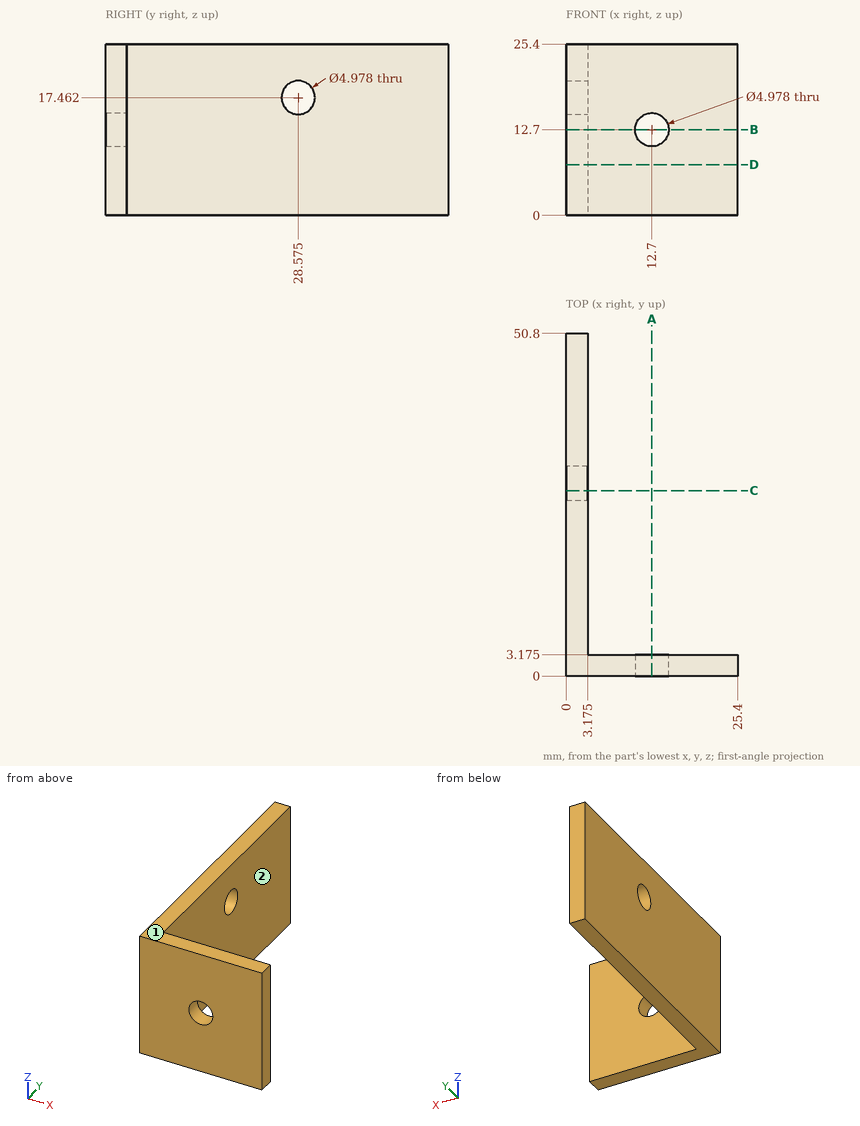
Design review of the part shown in the three views and the two pictorial views. Dimensions are in mm from the part's minimum x, y and z. A direction names the side the tool comes from. Coordinates: 2 decimals unless noted, no trailing zeros. Order: outer loops, then holes, each group sorted by start corner. A loop starts at its lowest first (then second) coordinate and runs counter-clockwise, first axis right, second up.
1) Clearance check with flat-ended pins moving along their axes: pin 1 (8 mm diameter, centred on x = 4, z = 15, fed in from +Y); pin 2 (1.5 mm diameter, centred on y = 36.5, z = 6, fed in from +X) (1 decimal); pin 3 (6 mm diameter, centred on x = 12.5, z = 10, fed in from +Y) (1 decimal). State where each tip first meets the part, or that it passes through.
2) For the marked faces 1 and 2, list the 3-axis set-ups (+Z, -Z, +X, -X, +Y, -Y) from which the entire face can be reached by the end or side of a thin tool; tool diameter is ignored.
3) Take a section at D-D, the plane z = 7.5. Give the boundary of the cut face in (x, y) (1 decimal).
4) Take a section at A-A, the plane x = 12.7. Give the boundary of the cut face in (y, z) (1 decimal).
5) Take a section at B-B, the plane z = 12.7. Give the boundary of the cut face in (x, y) (1 decimal).
6) Wall thickness on line 1 along Z through (x, y) = (12.7, 2.5); line 2 along X through (y, z) = (14.5, 7) (1 decimal): over which ranges is each line inside the solid? List them lowest first.
7) Take a section at C-C, the plane y = 27.5. Give the boundary of the cut face in (x, z) (1 decimal).
Returned:
1. pin 1: stops at y = 50.8
1. pin 2: stops at x = 3.2
1. pin 3: stops at y = 3.2
2. face 1: +Z, +X, -X, +Y, -Y
2. face 2: +Z, -Z, +X, +Y
3. outline: (0, 0) - (25.4, 0) - (25.4, 3.2) - (3.2, 3.2) - (3.2, 50.8) - (0, 50.8) - close
4. outline: (0, 0) - (3.2, 0) - (3.2, 10.2) - (0, 10.2) - close; (0, 15.2) - (3.2, 15.2) - (3.2, 25.4) - (0, 25.4) - close
5. outline: (0, 0) - (10.2, 0) - (10.2, 3.2) - (3.2, 3.2) - (3.2, 50.8) - (0, 50.8) - close; (15.2, 0) - (25.4, 0) - (25.4, 3.2) - (15.2, 3.2) - close
6. line 1: z = 0 to 10.21, 15.19 to 25.4
6. line 2: x = 0 to 3.2
7. outline: (0, 0) - (3.2, 0) - (3.2, 15.2) - (0, 15.2) - close; (0, 19.7) - (3.2, 19.7) - (3.2, 25.4) - (0, 25.4) - close
